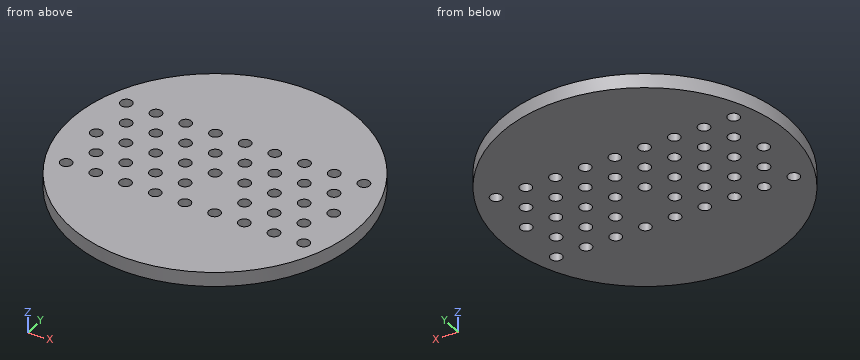
```python
from build123d import *

# Parameters (mm, degrees)
SKETCH_1_R           = 500
EXTRUDE_1_DEPTH      = 50
SKETCH_2_R           = 20
CUT_EXTRUDE_1_DEPTH  = 709.872343938
SKETCH_3_R           = 20
CUT_EXTRUDE_2_DEPTH  = 709.872343938
SKETCH_4_R           = 20
CUT_EXTRUDE_3_DEPTH  = 709.872343938
SKETCH_5_R           = 20
CUT_EXTRUDE_4_DEPTH  = 709.872343938
SKETCH_6_R           = 20
CUT_EXTRUDE_5_DEPTH  = 709.872343938
SKETCH_7_R           = 20
CUT_EXTRUDE_6_DEPTH  = 709.872343938
SKETCH_8_R           = 20
CUT_EXTRUDE_7_DEPTH  = 709.872343938
SKETCH_9_R           = 20
CUT_EXTRUDE_8_DEPTH  = 709.872343938
SKETCH_10_R          = 20
CUT_EXTRUDE_9_DEPTH  = 709.872343938
SKETCH_11_R          = 20
CUT_EXTRUDE_10_DEPTH = 709.872343938
SKETCH_12_R          = 20
CUT_EXTRUDE_11_DEPTH = 709.872343938
SKETCH_13_R          = 20
CUT_EXTRUDE_12_DEPTH = 709.872343938
SKETCH_14_R          = 20
CUT_EXTRUDE_13_DEPTH = 709.872343938
SKETCH_15_R          = 20
CUT_EXTRUDE_14_DEPTH = 709.872343938
SKETCH_16_R          = 20
CUT_EXTRUDE_15_DEPTH = 709.872343938
SKETCH_17_R          = 20
CUT_EXTRUDE_16_DEPTH = 709.872343938
SKETCH_18_R          = 20
CUT_EXTRUDE_17_DEPTH = 709.872343938
SKETCH_19_R          = 20
CUT_EXTRUDE_18_DEPTH = 709.872343938
SKETCH_20_R          = 20
CUT_EXTRUDE_19_DEPTH = 709.872343938
SKETCH_21_R          = 20
CUT_EXTRUDE_20_DEPTH = 709.872343938
SKETCH_22_R          = 20
CUT_EXTRUDE_21_DEPTH = 709.872343938
SKETCH_23_R          = 20
CUT_EXTRUDE_22_DEPTH = 709.872343938
SKETCH_24_R          = 20
CUT_EXTRUDE_23_DEPTH = 709.872343938
SKETCH_25_R          = 20
CUT_EXTRUDE_24_DEPTH = 709.872343938
SKETCH_26_R          = 20
CUT_EXTRUDE_25_DEPTH = 709.872343938
SKETCH_27_R          = 20
CUT_EXTRUDE_26_DEPTH = 709.872343938
SKETCH_28_R          = 20
CUT_EXTRUDE_27_DEPTH = 709.872343938
SKETCH_29_R          = 20
CUT_EXTRUDE_28_DEPTH = 709.872343938
SKETCH_30_R          = 20
CUT_EXTRUDE_29_DEPTH = 709.872343938
SKETCH_31_R          = 20
CUT_EXTRUDE_30_DEPTH = 709.872343938
SKETCH_32_R          = 20
CUT_EXTRUDE_31_DEPTH = 709.872343938
SKETCH_33_R          = 20
CUT_EXTRUDE_32_DEPTH = 709.872343938
SKETCH_34_R          = 20
CUT_EXTRUDE_33_DEPTH = 709.872343938
SKETCH_35_R          = 20
CUT_EXTRUDE_34_DEPTH = 709.872343938
SKETCH_36_R          = 20
CUT_EXTRUDE_35_DEPTH = 709.872343938
SKETCH_37_R          = 20
CUT_EXTRUDE_36_DEPTH = 709.872343938
SKETCH_38_R          = 20
CUT_EXTRUDE_37_DEPTH = 709.872343938
SKETCH_39_R          = 20
CUT_EXTRUDE_38_DEPTH = 709.872343938
SKETCH_40_R          = 20
CUT_EXTRUDE_39_DEPTH = 709.872343938
SKETCH_41_R          = 20
CUT_EXTRUDE_40_DEPTH = 709.872343938
SKETCH_42_R          = 20
CUT_EXTRUDE_41_DEPTH = 709.872343938
SKETCH_43_R          = 20
CUT_EXTRUDE_42_DEPTH = 709.872343938


with BuildPart() as part:
    # 草图1 → 凸台-拉伸1 (new body)
    with BuildSketch(Plane.XY):
        Circle(SKETCH_1_R)
    extrude(amount=EXTRUDE_1_DEPTH)

    # 草图2 → 切除-拉伸1 (cut, through all)
    with BuildSketch(Plane.XY):
        with Locations((-400, 0)):
            Circle(SKETCH_2_R)
    extrude(amount=CUT_EXTRUDE_1_DEPTH, mode=Mode.SUBTRACT)

    # 草图3 → 切除-拉伸2 (cut, through all)
    with BuildSketch(Plane.XY):
        with Locations((-300, 0)):
            Circle(SKETCH_3_R)
    extrude(amount=CUT_EXTRUDE_2_DEPTH, mode=Mode.SUBTRACT)

    # 草图4 → 切除-拉伸3 (cut, through all)
    with BuildSketch(Plane.XY):
        with Locations((-200, 0)):
            Circle(SKETCH_4_R)
    extrude(amount=CUT_EXTRUDE_3_DEPTH, mode=Mode.SUBTRACT)

    # 草图5 → 切除-拉伸4 (cut, through all)
    with BuildSketch(Plane.XY):
        with Locations((-100, 0)):
            Circle(SKETCH_5_R)
    extrude(amount=CUT_EXTRUDE_4_DEPTH, mode=Mode.SUBTRACT)

    # 草图6 → 切除-拉伸5 (cut, through all)
    with BuildSketch(Plane.XY):
        Circle(SKETCH_6_R)
    extrude(amount=CUT_EXTRUDE_5_DEPTH, mode=Mode.SUBTRACT)

    # 草图7 → 切除-拉伸6 (cut, through all)
    with BuildSketch(Plane.XY):
        with Locations((100, 0)):
            Circle(SKETCH_7_R)
    extrude(amount=CUT_EXTRUDE_6_DEPTH, mode=Mode.SUBTRACT)

    # 草图8 → 切除-拉伸7 (cut, through all)
    with BuildSketch(Plane.XY):
        with Locations((200, 0)):
            Circle(SKETCH_8_R)
    extrude(amount=CUT_EXTRUDE_7_DEPTH, mode=Mode.SUBTRACT)

    # 草图9 → 切除-拉伸8 (cut, through all)
    with BuildSketch(Plane.XY):
        with Locations((300, 0)):
            Circle(SKETCH_9_R)
    extrude(amount=CUT_EXTRUDE_8_DEPTH, mode=Mode.SUBTRACT)

    # 草图10 → 切除-拉伸9 (cut, through all)
    with BuildSketch(Plane.XY):
        with Locations((400, 0)):
            Circle(SKETCH_10_R)
    extrude(amount=CUT_EXTRUDE_9_DEPTH, mode=Mode.SUBTRACT)

    # 草图11 → 切除-拉伸10 (cut, through all)
    with BuildSketch(Plane.XY):
        with Locations((-350, 86.6)):
            Circle(SKETCH_11_R)
    extrude(amount=CUT_EXTRUDE_10_DEPTH, mode=Mode.SUBTRACT)

    # 草图12 → 切除-拉伸11 (cut, through all)
    with BuildSketch(Plane.XY):
        with Locations((-250, 86.6)):
            Circle(SKETCH_12_R)
    extrude(amount=CUT_EXTRUDE_11_DEPTH, mode=Mode.SUBTRACT)

    # 草图13 → 切除-拉伸12 (cut, through all)
    with BuildSketch(Plane.XY):
        with Locations((-150, 86.6)):
            Circle(SKETCH_13_R)
    extrude(amount=CUT_EXTRUDE_12_DEPTH, mode=Mode.SUBTRACT)

    # 草图14 → 切除-拉伸13 (cut, through all)
    with BuildSketch(Plane.XY):
        with Locations((-50, 86.6)):
            Circle(SKETCH_14_R)
    extrude(amount=CUT_EXTRUDE_13_DEPTH, mode=Mode.SUBTRACT)

    # 草图15 → 切除-拉伸14 (cut, through all)
    with BuildSketch(Plane.XY):
        with Locations((50, 86.6)):
            Circle(SKETCH_15_R)
    extrude(amount=CUT_EXTRUDE_14_DEPTH, mode=Mode.SUBTRACT)

    # 草图16 → 切除-拉伸15 (cut, through all)
    with BuildSketch(Plane.XY):
        with Locations((150, 86.6)):
            Circle(SKETCH_16_R)
    extrude(amount=CUT_EXTRUDE_15_DEPTH, mode=Mode.SUBTRACT)

    # 草图17 → 切除-拉伸16 (cut, through all)
    with BuildSketch(Plane.XY):
        with Locations((250, 86.6)):
            Circle(SKETCH_17_R)
    extrude(amount=CUT_EXTRUDE_16_DEPTH, mode=Mode.SUBTRACT)

    # 草图18 → 切除-拉伸17 (cut, through all)
    with BuildSketch(Plane.XY):
        with Locations((350, 86.6)):
            Circle(SKETCH_18_R)
    extrude(amount=CUT_EXTRUDE_17_DEPTH, mode=Mode.SUBTRACT)

    # 草图19 → 切除-拉伸18 (cut, through all)
    with BuildSketch(Plane.XY):
        with Locations((-400, 173.2)):
            Circle(SKETCH_19_R)
    extrude(amount=CUT_EXTRUDE_18_DEPTH, mode=Mode.SUBTRACT)

    # 草图20 → 切除-拉伸19 (cut, through all)
    with BuildSketch(Plane.XY):
        with Locations((-300, 173.2)):
            Circle(SKETCH_20_R)
    extrude(amount=CUT_EXTRUDE_19_DEPTH, mode=Mode.SUBTRACT)

    # 草图21 → 切除-拉伸20 (cut, through all)
    with BuildSketch(Plane.XY):
        with Locations((-200, 173.2)):
            Circle(SKETCH_21_R)
    extrude(amount=CUT_EXTRUDE_20_DEPTH, mode=Mode.SUBTRACT)

    # 草图22 → 切除-拉伸21 (cut, through all)
    with BuildSketch(Plane.XY):
        with Locations((-100, 173.2)):
            Circle(SKETCH_22_R)
    extrude(amount=CUT_EXTRUDE_21_DEPTH, mode=Mode.SUBTRACT)

    # 草图23 → 切除-拉伸22 (cut, through all)
    with BuildSketch(Plane.XY):
        with Locations((0, 173.2)):
            Circle(SKETCH_23_R)
    extrude(amount=CUT_EXTRUDE_22_DEPTH, mode=Mode.SUBTRACT)

    # 草图24 → 切除-拉伸23 (cut, through all)
    with BuildSketch(Plane.XY):
        with Locations((100, 173.2)):
            Circle(SKETCH_24_R)
    extrude(amount=CUT_EXTRUDE_23_DEPTH, mode=Mode.SUBTRACT)

    # 草图25 → 切除-拉伸24 (cut, through all)
    with BuildSketch(Plane.XY):
        with Locations((200, 173.2)):
            Circle(SKETCH_25_R)
    extrude(amount=CUT_EXTRUDE_24_DEPTH, mode=Mode.SUBTRACT)

    # 草图26 → 切除-拉伸25 (cut, through all)
    with BuildSketch(Plane.XY):
        with Locations((300, 173.2)):
            Circle(SKETCH_26_R)
    extrude(amount=CUT_EXTRUDE_25_DEPTH, mode=Mode.SUBTRACT)

    # 草图27 → 切除-拉伸26 (cut, through all)
    with BuildSketch(Plane.XY):
        with Locations((400, 173.2)):
            Circle(SKETCH_27_R)
    extrude(amount=CUT_EXTRUDE_26_DEPTH, mode=Mode.SUBTRACT)

    # 草图28 → 切除-拉伸27 (cut, through all)
    with BuildSketch(Plane.XY):
        with Locations((-350, -86.6)):
            Circle(SKETCH_28_R)
    extrude(amount=CUT_EXTRUDE_27_DEPTH, mode=Mode.SUBTRACT)

    # 草图29 → 切除-拉伸28 (cut, through all)
    with BuildSketch(Plane.XY):
        with Locations((-250, -86.6)):
            Circle(SKETCH_29_R)
    extrude(amount=CUT_EXTRUDE_28_DEPTH, mode=Mode.SUBTRACT)

    # 草图30 → 切除-拉伸29 (cut, through all)
    with BuildSketch(Plane.XY):
        with Locations((-150, -86.6)):
            Circle(SKETCH_30_R)
    extrude(amount=CUT_EXTRUDE_29_DEPTH, mode=Mode.SUBTRACT)

    # 草图31 → 切除-拉伸30 (cut, through all)
    with BuildSketch(Plane.XY):
        with Locations((-50, -86.6)):
            Circle(SKETCH_31_R)
    extrude(amount=CUT_EXTRUDE_30_DEPTH, mode=Mode.SUBTRACT)

    # 草图32 → 切除-拉伸31 (cut, through all)
    with BuildSketch(Plane.XY):
        with Locations((150, -86.6)):
            Circle(SKETCH_32_R)
    extrude(amount=CUT_EXTRUDE_31_DEPTH, mode=Mode.SUBTRACT)

    # 草图33 → 切除-拉伸32 (cut, through all)
    with BuildSketch(Plane.XY):
        with Locations((250, -86.6)):
            Circle(SKETCH_33_R)
    extrude(amount=CUT_EXTRUDE_32_DEPTH, mode=Mode.SUBTRACT)

    # 草图34 → 切除-拉伸33 (cut, through all)
    with BuildSketch(Plane.XY):
        with Locations((350, -86.6)):
            Circle(SKETCH_34_R)
    extrude(amount=CUT_EXTRUDE_33_DEPTH, mode=Mode.SUBTRACT)

    # 草图35 → 切除-拉伸34 (cut, through all)
    with BuildSketch(Plane.XY):
        with Locations((-400, -173.2)):
            Circle(SKETCH_35_R)
    extrude(amount=CUT_EXTRUDE_34_DEPTH, mode=Mode.SUBTRACT)

    # 草图36 → 切除-拉伸35 (cut, through all)
    with BuildSketch(Plane.XY):
        with Locations((-300, -173.2)):
            Circle(SKETCH_36_R)
    extrude(amount=CUT_EXTRUDE_35_DEPTH, mode=Mode.SUBTRACT)

    # 草图37 → 切除-拉伸36 (cut, through all)
    with BuildSketch(Plane.XY):
        with Locations((-200, -173.2)):
            Circle(SKETCH_37_R)
    extrude(amount=CUT_EXTRUDE_36_DEPTH, mode=Mode.SUBTRACT)

    # 草图38 → 切除-拉伸37 (cut, through all)
    with BuildSketch(Plane.XY):
        with Locations((-100, -173.2)):
            Circle(SKETCH_38_R)
    extrude(amount=CUT_EXTRUDE_37_DEPTH, mode=Mode.SUBTRACT)

    # 草图39 → 切除-拉伸38 (cut, through all)
    with BuildSketch(Plane.XY):
        with Locations((0, -173.2)):
            Circle(SKETCH_39_R)
    extrude(amount=CUT_EXTRUDE_38_DEPTH, mode=Mode.SUBTRACT)

    # 草图40 → 切除-拉伸39 (cut, through all)
    with BuildSketch(Plane.XY):
        with Locations((100, -173.2)):
            Circle(SKETCH_40_R)
    extrude(amount=CUT_EXTRUDE_39_DEPTH, mode=Mode.SUBTRACT)

    # 草图41 → 切除-拉伸40 (cut, through all)
    with BuildSketch(Plane.XY):
        with Locations((200, -173.2)):
            Circle(SKETCH_41_R)
    extrude(amount=CUT_EXTRUDE_40_DEPTH, mode=Mode.SUBTRACT)

    # 草图42 → 切除-拉伸41 (cut, through all)
    with BuildSketch(Plane.XY):
        with Locations((300, -173.2)):
            Circle(SKETCH_42_R)
    extrude(amount=CUT_EXTRUDE_41_DEPTH, mode=Mode.SUBTRACT)

    # 草图43 → 切除-拉伸42 (cut, through all)
    with BuildSketch(Plane.XY):
        with Locations((400, -173.2)):
            Circle(SKETCH_43_R)
    extrude(amount=CUT_EXTRUDE_42_DEPTH, mode=Mode.SUBTRACT)


solid = part.part
```
For this review, take the finished solid that the model builds, in its own axes (mm). Round coordinates to 2 decimals unless told otherwise and drop trailing zeros. Write each loop counter-clockwise with the first axis right and the second up, starting at its lowest first coordinate (ties: lowest second). Pieces come first, ordered by that corner, then holes. Notation, with made-up numbers: (2, 27.5) -> (39, 27.5) arc R12 ccw to (39, 40.5) -> close; hole circle Ø6 at (14.5, 84). An arc over 180 degrees is marked (long way). One line per question, with ' | ' between items. Start each with the question number.
(1) Add section C-C, the plane y = -86.6. Give the number of separate pieces and of enclosed holes in the cut face, plus the area to 3 significant figures.
(2) Add section B-B, the plane x = -50. Write out the cut boundary in (y, z).
(3) Add section A-A, the plane x = -400. Write out the cut boundary in (y, z), plus the area to 3 significant figures.
(4) For line 1 along Y through (x, z) = (0, 36.5); line 2 along Y through (x, z) = (-350, 17); line 3 along Y through (x, z) = (-216, 5.5), list the stretches that pass through material, from the lowest coordinate up. Write a range as from..to.
(5) Insertion check: P1, Ø1.5, axis at y = 277, z = 8, coming from the +X side; P2, Ø24, axis at x = -350, y = 86.6, coming from the +Z side; P3, Ø4, axis at y = -172, z = 44.5, coming from the -X side; P4, Ø3, axis at y = 190.5, z = 40, coming from the -X side. Each pin has a flat end and moves straight along its axis. Give the tip position at first contact, or say it passes through.
Answer list:
1) separate pieces: 8 | enclosed holes: 0 | area: 35,200 mm²
2) outline: (-497.49, 0) -> (-106.6, 0) -> (-106.6, 50) -> (-497.49, 50) -> close; (-66.6, 0) -> (66.6, 0) -> (66.6, 50) -> (-66.6, 50) -> close; (106.6, 0) -> (497.49, 0) -> (497.49, 50) -> (106.6, 50) -> close
3) outline: (-300, 0) -> (-193.2, 0) -> (-193.2, 50) -> (-300, 50) -> close; (-153.2, 0) -> (-20, 0) -> (-20, 50) -> (-153.2, 50) -> close; (20, 0) -> (153.2, 0) -> (153.2, 50) -> (20, 50) -> close; (193.2, 0) -> (300, 0) -> (300, 50) -> (193.2, 50) -> close | area: 24,000 mm²
4) line 1: -500..-193.2, -153.2..-20, 20..153.2, 193.2..500 | line 2: -357.07..-106.6, -66.6..66.6, 106.6..357.07 | line 3: -450.94..-185.2, -161.2..-12, 12..161.2, 185.2..450.94
5) P1: x = 416.76 | P2: through | P3: x = -470.21 | P4: x = -462.9
